Model file for the job. Use its own axes, mm. A direction names the side the tool comes from. Give positions to 0.01 mm unless a question says otherwise; leave off trailing zeros. Write each loop counter-clockwise with the first axis right and the second up, starting at its lowest first coordinate (ties: lowest second). Pieces come first, ordered by that corner, then holes.
```python
from build123d import *

# Parameters (mm, degrees)
CROQUIS1_R              = 1.75
SALIENTE_EXTRUIR1_DEPTH = 1.5875
REDONDEO1_R             = 8


with BuildPart() as part:
    # Croquis1 → Saliente-Extruir1 (new, symmetric)
    with BuildSketch(Plane(origin=(0, 0, 0), x_dir=(1, 0, 0), z_dir=(0, 1, 0))):
        with BuildLine():
            Line((8.1, 0), (-8.1, 0))
            Line((-8.1, 0), (-8.1, -12))
            Line((-8.1, -12), (-20, -12))
            Line((-20, -12), (-20, 5))
            Line((-20, 5), (-19, 5))
            Line((-19, 5), (-19, 71.5))
            ThreePointArc((-19, 71.5), (-17.974873734, 73.974873734), (-15.5, 75))
            Line((-15.5, 75), (-14.5, 75))
            ThreePointArc((-14.5, 75), (-12.025126266, 73.974873734), (-11, 71.5))
            Line((-11, 71.5), (-11, 5))
            Line((-11, 5), (11, 5))
            Line((11, 5), (11, 71.5))
            ThreePointArc((11, 71.5), (12.025126266, 73.974873734), (14.5, 75))
            Line((14.5, 75), (15.5, 75))
            ThreePointArc((15.5, 75), (17.974873734, 73.974873734), (19, 71.5))
            Line((19, 71.5), (19, 5))
            Line((19, 5), (20, 5))
            Line((20, 5), (20, -12))
            Line((20, -12), (8.1, -12))
            Line((8.1, -12), (8.1, 0))
        make_face()
        with Locations(Location((-13, -6, 0), (0, 0, 270))):
            Circle(CROQUIS1_R, mode=Mode.SUBTRACT)
        with Locations(Location((13, -6, 0), (0, 0, 270))):
            Circle(CROQUIS1_R, mode=Mode.SUBTRACT)
    extrude(amount=SALIENTE_EXTRUIR1_DEPTH, both=True)

    # Redondeo1
    redondeo1_edges = [part.edges().sort_by_distance(p)[0] for p in [
        (-11, 0, -5),
        (11, 0, -5),
    ]]
    fillet(redondeo1_edges, radius=REDONDEO1_R)


solid = part.part
```
1. Which spindle directions (+Z, -Z, +X, -X, +Y, -Y) get a long thin tool onto all of the face, cutting with end or side? Do faces 1 (the flat face through (19, 0, -39)), 2 (the flat face through (8.1, 0, 6)), 3 (the cylindrical face through (12, 0.02, -73.95)). Say none if no direction does.
Calculated:
face 1: -Z, +X, +Y, -Y
face 2: +Z, +Y, -Y
face 3: -Z, +Y, -Y
2. Pull direction Z, two halves, no side cores. Call faces 4 (the cylindrical face through (14.735, -0.022, 5.772)), 5 (the cylindrical face through (-11.265, -0.022, 5.772)), 6 (the flat face through (0, 0, 0)), 7 (the flat face through (20, 0, 3)): +Z half, -Z half, draft (parallel to the pull), parting line (faces both ways), or undercut.
Calculated:
face 4: undercut
face 5: undercut
face 6: +Z half
face 7: draft
3. Slice it at D-D, the plane x = -13. Write the cut outline in (y, z), and give its area (3 significant figures).
Calculated:
outline: (-1.59, -74.66) - (1.59, -74.66) - (1.59, 4.25) - (-1.59, 4.25) - close; (-1.59, 7.75) - (1.59, 7.75) - (1.59, 12) - (-1.59, 12) - close
area: 264 mm2
4. Slice it at C-C, the plane z = 6. Write the cut outline in (x, y).
Calculated:
outline: (-20, -1.59) - (-14.75, -1.59) - (-14.75, 1.59) - (-20, 1.59) - close; (-11.25, -1.59) - (-8.1, -1.59) - (-8.1, 1.59) - (-11.25, 1.59) - close; (8.1, -1.59) - (11.25, -1.59) - (11.25, 1.59) - (8.1, 1.59) - close; (14.75, -1.59) - (20, -1.59) - (20, 1.59) - (14.75, 1.59) - close
5. Slice it at B-B, the plane y = 0.55. Write the cut outline in (x, z).
Calculated:
outline: (-20, -5) - (-19, -5) - (-19, -71.5) arc R3.5 ccw to (-15.5, -75) - (-14.5, -75) arc R3.5 ccw to (-11, -71.5) - (-11, -13) arc R8 cw to (-3, -5) - (3, -5) arc R8 cw to (11, -13) - (11, -71.5) arc R3.5 ccw to (14.5, -75) - (15.5, -75) arc R3.5 ccw to (19, -71.5) - (19, -5) - (20, -5) - (20, 12) - (8.1, 12) - (8.1, 0) - (-8.1, 0) - (-8.1, 12) - (-20, 12) - close; hole circle Ø3.5 at (-13, 6); hole circle Ø3.5 at (13, 6)
6. Slice it at A-A, the plane z = -25. Write the cut outline in (x, y), and give its area (3 significant figures).
Calculated:
outline: (-19, -1.59) - (-11, -1.59) - (-11, 1.59) - (-19, 1.59) - close; (11, -1.59) - (19, -1.59) - (19, 1.59) - (11, 1.59) - close
area: 50.8 mm2
7. Pin check, flat tips, straight feed: P1, Ø0.8, axis at x = -19.5, y = -0.5, coming from the -Z side; P2, Ø1.6, axis at y = 0.5, z = -45, coming from the -X side. Stop position of each tip, or through.
Calculated:
P1: stops at z = -5
P2: stops at x = -19
8. Probe probe 1 along X at (y, z) = (-0.6, 6); probe 2 along X at (y, z) = (0.2, -63.5); probe 3 along X at (y, z) = (-0.1, -11). List the from-to ranges inside material, lowest first.
Calculated:
probe 1: x = -20 to -14.75, -11.25 to -8.1, 8.1 to 11.25, 14.75 to 20
probe 2: x = -19 to -11, 11 to 19
probe 3: x = -19 to -10.75, 10.75 to 19
